Verification items for this drawing (mm, ordinates from the low corner). A direction names the side the tool comes from. Coordinates: 2 decimals unless noted, no trailing zeros. Order: outer loops, then holes, each group sorted by start corner. A loop starts at its lowest first (then second) coordinate and runs counter-clockwise, first axis right, second up. Notation, with made-up numbers: (-6.5, 56) -> (10.5, 56) arc R17 ccw to (10.5, 63) -> close; hole circle Ø4 at (-23, 33.25). An arc over 180 degrees is marked (long way). Write each question's results on one line, items separated by ' | '. Start each with the question number.
(1) Draft check along Y on the marked faces 1, 2, 3 and 4. Enter one of: +Y half, -Y half, draft (parallel to the pull), parting line (faces both ways), or undercut.
(2) Set-up check for the marked faces 5 and 6: record each of +Z, -Z, +X, -X, +Y, -Y from which the full face is reachable in a straight line by a thin tool's end or side.
(3) Cross-section at C-C on z = 4. Enter the section's corners in (x, y).
(4) Cross-section at A-A on z = 20. Enter the section's corners in (x, y).
(5) Thickness scan on probe 1 along X at (y, z) = (69.5, 39); probe 2 along Z at (x, y) = (82.5, 90); probe 3 along Y at (x, z) = (90, 11.5). Record the ranges inside material, lowest first. Write a range as [from, to].
(6) Cross-section at D-D on y = 91. Enter the section's corners in (x, z), and give its area (3 significant figures).
(7) Go/stop test with flat-tipped pins: pin 1 (10 mm diameter, centred on x = 78.5, y = 49, fed in from +Z); pin 2 (1 mm diameter, centred on x = 32, z = 22.5, fed in from -Y); pin 3 (6 mm diameter, centred on x = 17.5, z = 18, fed in from -Y). Record where each tip stops, or that it passes through.
(8) Cross-section at B-B on y = 74. Enter the section's corners in (x, z), and give its area (3 significant figures).
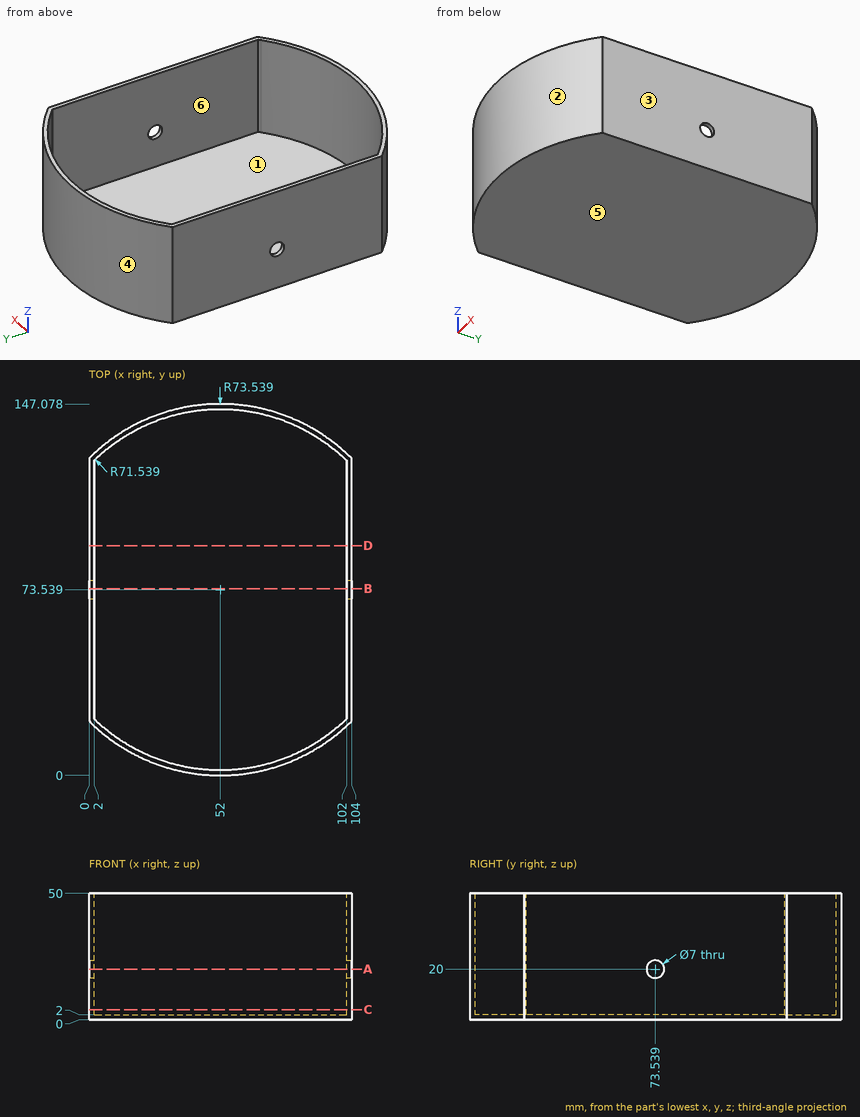
Results are:
1) face 1: undercut | face 2: -Y half | face 3: draft | face 4: +Y half
2) face 5: -Z, +X, -X, +Y, -Y | face 6: +Z
3) outline: (0, 21.54) arc R73.54 ccw to (104, 21.54) -> (104, 125.54) arc R73.54 ccw to (0, 125.54) -> close; hole (2, 22.37) arc R71.54 ccw to (102, 22.37) -> (102, 124.7) arc R71.54 ccw to (2, 124.7) -> close
4) outline: (0, 21.54) arc R73.54 ccw to (104, 21.54) -> (104, 70.04) -> (102, 70.04) -> (102, 22.37) arc R71.54 cw to (2, 22.37) -> (2, 70.04) -> (0, 70.04) -> close; (0, 77.04) -> (2, 77.04) -> (2, 124.7) arc R71.54 cw to (102, 124.7) -> (102, 77.04) -> (104, 77.04) -> (104, 125.54) arc R73.54 ccw to (0, 125.54) -> close
5) probe 1: x = [0, 2], [102, 104] | probe 2: z = [0, 2] | probe 3: y = [10.58, 12.93], [134.15, 136.5]
6) outline: (0, 0) -> (104, 0) -> (104, 50) -> (102, 50) -> (102, 2) -> (2, 2) -> (2, 50) -> (0, 50) -> close | area: 400 mm2
7) pin 1: stops at z = 2 | pin 2: stops at y = 2.63 | pin 3: stops at y = 7.09
8) outline: (0, 0) -> (104, 0) -> (104, 16.53) -> (102, 16.53) -> (102, 2) -> (2, 2) -> (2, 16.53) -> (0, 16.53) -> close; (0, 23.47) -> (2, 23.47) -> (2, 50) -> (0, 50) -> close; (102, 23.47) -> (104, 23.47) -> (104, 50) -> (102, 50) -> close | area: 372 mm2
